Design review of the part built by this model. Coordinates are the model's own, in mm. A direction names the side the tool comes from. Coordinates: 2 decimals unless noted, no trailing zeros.
Q1. Add section A-A on x = 18.5. Give the number of separate pieces and of enclosed holes in the cut face, and give its area (3 significant figures).
Q2. Draft analysis for pull direction X (two halves, no side actions). For faces 1 (the face through (-26.453, -25.269, 5.07)), 2 (the face through (14, 1, 10)), 3 (the face through (60, 1, 5)), state which applies: released by +X, released by -X, zero draft, split by the parting line, or undercut.
Q3. Machinability: for faces 4 (the face through (15.894, 29.056, 5.07)), 5 (the face through (-60, -1, 5)), which of the approach directions +Z, -Z, +X, -X, +Y, -Y give a long, thin tool a straight path to every point of the face, cutting with its end or side? Answer none if there is none.
Q4. Wall thickness on probe 1 along Y at (x, z) = (-21, 3.5); probe 2 along Y at (x, z) = (-22, 8); probe 3 along Y at (x, z) = (-8, 8): over which ranges is each line inside the solid? List them lowest first.
```python
from build123d import *

# Parameters (mm, degrees)
BOSS_EXTRUDE1_DEPTH = 10
CUT_EXTRUDE32_DEPTH = 10


with BuildPart() as part:
    # Sketch1 → Boss-Extrude1 (new body)
    with BuildSketch(Plane.XY):
        with BuildLine():
            Line((-50, 60), (50, 60))
            ThreePointArc((50, 60), (57.071067812, 57.071067812), (60, 50))
            Line((60, 50), (60, -50))
            ThreePointArc((60, -50), (57.071067812, -57.071067812), (50, -60))
            Line((50, -60), (-50, -60))
            ThreePointArc((-50, -60), (-57.071067812, -57.071067812), (-60, -50))
            Line((-60, -50), (-60, 50))
            ThreePointArc((-60, 50), (-57.071067812, 57.071067812), (-50, 60))
        make_face()
    extrude(amount=BOSS_EXTRUDE1_DEPTH)

    # Sketch2 → Cut-Extrude32 (cut)
    with BuildSketch(Plane.XY.offset(10)):
        with BuildLine():
            Line((22.179487179, 34.806690705), (9.429086538, 23.141025641))
            add(Edge.make_bspline(
                [(9.429086538, 23.141025641), (8.882914048, 23.91145872), (7.834339031, 25.390582792), (6.134708299, 27.371164786), (4.442752271, 29.06074862), (2.742796004, 30.452275993), (1.019771731, 31.537292342), (-0.723329628, 32.305495903), (-2.476625945, 32.793850197), (-3.654570423, 32.854662056), (-4.234775641, 32.884615385)],
                knots=[0, 0, 0, 0, 1.299362458, 2.494594718, 3.587462134, 4.587049575, 5.512617175, 6.380583204, 7.202344345, 8, 8, 8, 8], degree=3))
            add(Edge.make_bspline(
                [(-4.234775641, 32.884615385), (-4.775974426, 32.865635582), (-5.820887089, 32.828990568), (-7.31048761, 32.464741869), (-8.632976167, 31.836102106), (-9.787062069, 31.01410273), (-10.701268375, 30.023784052), (-11.431191215, 28.98519439), (-11.842199109, 27.838826287), (-11.896295835, 27.05145443), (-11.923076923, 26.661658654)],
                knots=[0, 0, 0, 0, 1.185010067, 2.2879431, 3.333075148, 4.379039566, 5.372662701, 6.27520591, 7.14612461, 8, 8, 8, 8], degree=3))
            add(Edge.make_bspline(
                [(-11.923076923, 26.661658654), (-11.906294573, 26.266241849), (-11.872497251, 25.469927355), (-11.546061132, 24.302829291), (-11.054028691, 23.162438622), (-10.583871606, 22.468228557), (-10.343549679, 22.11338141)],
                knots=[0, 0, 0, 0, 0.967525499, 1.948461899, 2.951351359, 4, 4, 4, 4], degree=3))
            add(Edge.make_bspline(
                [(-10.343549679, 22.11338141), (-10.125071051, 21.837562436), (-9.622162103, 21.202663585), (-8.663217741, 20.197082772), (-7.458985017, 18.965158257), (-5.96312252, 17.549252313), (-4.237727617, 15.898443424), (-2.202826025, 14.077625518), (0.083008913, 12.030409979), (1.707727428, 10.604803211), (2.559094551, 9.857772436)],
                knots=[0, 0, 0, 0, 0.473873513, 1.090794244, 1.870441696, 2.795289791, 3.865433203, 5.087734844, 6.473946851, 8, 8, 8, 8], degree=3))
            add(Edge.make_bspline(
                [(2.559094551, 9.857772436), (3.358225064, 9.166165286), (4.874808752, 7.853638601), (7.032606174, 5.990717711), (8.92895073, 4.31469321), (10.591467834, 2.85071864), (11.994955347, 1.583433555), (13.145313536, 0.506780349), (14.056592075, -0.358280522), (14.574600568, -0.880777815), (14.795673077, -1.103766026)],
                knots=[0, 0, 0, 0, 1.543621617, 2.929473131, 4.163658386, 5.240097082, 6.164993805, 6.925417477, 7.541396219, 8, 8, 8, 8], degree=3))
            add(Edge.make_bspline(
                [(14.795673077, -1.103766026), (15.634376084, -2.011422303), (17.246657803, -3.756256423), (19.342055672, -6.460200571), (21.066635897, -9.099801404), (22.400803862, -11.724727295), (23.40842117, -14.372850698), (24.118804721, -17.109116699), (24.544258155, -19.96211756), (24.59149342, -21.908942364), (24.615384615, -22.893629808)],
                knots=[0, 0, 0, 0, 1.206664779, 2.319633467, 3.337109185, 4.282041471, 5.190008762, 6.099243693, 7.03861361, 8, 8, 8, 8], degree=3))
            add(Edge.make_bspline(
                [(24.615384615, -22.893629808), (24.598379474, -23.853086961), (24.565014754, -25.735577605), (24.156360918, -28.490322254), (23.573644532, -31.126732441), (22.672662774, -33.616120296), (21.574551543, -35.999348361), (20.197910517, -38.239293521), (18.581234396, -40.358624937), (16.728275333, -42.319456968), (14.67868258, -44.098776126), (12.480299564, -45.682768067), (10.111629387, -46.990555178), (7.592909595, -48.06742458), (4.925488401, -48.896843793), (2.112543508, -49.509861892), (-0.850227675, -49.877785692), (-2.876213304, -49.91624776), (-3.911258013, -49.935897436)],
                knots=[0, 0, 0, 0, 1.043214005, 2.046824704, 3.02475056, 3.976699089, 4.921714032, 5.875962561, 6.831408892, 7.817874052, 8.806269674, 9.781291748, 10.760897367, 11.74438705, 12.757449933, 13.795994037, 14.874007457, 16, 16, 16, 16], degree=3))
            add(Edge.make_bspline(
                [(-3.911258013, -49.935897436), (-4.723759295, -49.921483122), (-6.332977804, -49.892934513), (-8.704722601, -49.659858889), (-10.994910313, -49.283699628), (-13.200961249, -48.74455104), (-15.332814058, -48.061376655), (-17.390556291, -47.226905315), (-19.359982672, -46.228203026), (-21.255994813, -45.085807078), (-23.069375756, -43.759334902), (-24.82305499, -42.275905787), (-26.499613308, -40.612703931), (-28.107102878, -38.773662739), (-29.635238535, -36.753574491), (-31.134041642, -34.580572653), (-32.53690088, -32.214329262), (-33.403509434, -30.554390381), (-33.846153846, -29.706530449)],
                knots=[0, 0, 0, 0, 1.016823716, 2.013894106, 2.979844003, 3.91962641, 4.853723003, 5.779685073, 6.695824784, 7.614987388, 8.547259901, 9.504950863, 10.487499108, 11.500346958, 12.559593716, 13.656357062, 14.802919212, 16, 16, 16, 16], degree=3))
            Line((-33.846153846, -29.706530449), (-18.850160256, -20.705128205))
            add(Edge.make_bspline(
                [(-18.850160256, -20.705128205), (-18.296478254, -21.667560008), (-17.235022533, -23.512624029), (-15.436286582, -25.991701389), (-13.593573429, -28.114620785), (-11.664281196, -29.843859481), (-9.671869355, -31.202539621), (-7.606714094, -32.173546708), (-5.467364474, -32.774598996), (-4.010136703, -32.848001363), (-3.283253205, -32.884615385)],
                knots=[0, 0, 0, 0, 1.283663364, 2.460892379, 3.537111102, 4.529833553, 5.449777664, 6.316464042, 7.160231139, 8, 8, 8, 8], degree=3))
            add(Edge.make_bspline(
                [(-3.283253205, -32.884615385), (-2.543908622, -32.854714389), (-1.109472453, -32.796702103), (0.938001622, -32.26086011), (2.81520338, -31.41954887), (4.437842715, -30.219113746), (5.811791397, -28.83362916), (6.825844389, -27.292214207), (7.462879318, -25.624440438), (7.530229355, -24.465895073), (7.564102564, -23.883213141)],
                knots=[0, 0, 0, 0, 1.13588714, 2.203786484, 3.234766741, 4.283437687, 5.291419208, 6.222934724, 7.106237994, 8, 8, 8, 8], degree=3))
            add(Edge.make_bspline(
                [(7.564102564, -23.883213141), (7.532822042, -23.341122423), (7.469278655, -22.239917025), (7.001237654, -20.602601675), (6.26954681, -18.966030942), (5.403904944, -17.62367135), (4.523005953, -16.499750052), (3.68066783, -15.525923088), (2.654922822, -14.450014779), (1.448371765, -13.270671713), (0.076956347, -11.977511836), (-1.460478671, -10.570661777), (-3.181538547, -9.062514205), (-4.397987064, -8.035178979), (-5.034054487, -7.497996795)],
                knots=[0, 0, 0, 0, 0.916159276, 1.861089862, 2.860218735, 3.940849679, 4.552606315, 5.27541173, 6.11797699, 7.06649574, 8.129236253, 9.306560635, 10.591630461, 12, 12, 12, 12], degree=3))
            add(Edge.make_bspline(
                [(-5.034054487, -7.497996795), (-6.243243975, -6.474906536), (-8.564044597, -4.511286663), (-11.84363032, -1.611081927), (-14.798830707, 1.099425143), (-17.404121473, 3.653742339), (-19.692698053, 6.004697341), (-21.649061212, 8.171385505), (-23.251719411, 10.170519868), (-24.938171589, 12.538360741), (-26.540638342, 15.423737543), (-27.925624358, 18.895180326), (-28.824144829, 22.366182634), (-28.924811551, 24.696422404), (-28.974358974, 25.843349359)],
                knots=[0, 0, 0, 0, 1.345494975, 2.582412109, 3.71882943, 4.751509156, 5.681369928, 6.505683931, 7.230279997, 7.856715994, 8.973648664, 10.023341002, 11.027102913, 12, 12, 12, 12], degree=3))
            add(Edge.make_bspline(
                [(-28.974358974, 25.843349359), (-28.953752267, 26.656688395), (-28.91315484, 28.259053664), (-28.551019527, 30.61509832), (-28.009794504, 32.888483451), (-27.223780391, 35.070914712), (-26.203628979, 37.159658519), (-24.964694716, 39.164940152), (-23.487739299, 41.068303453), (-21.823310254, 42.868486626), (-19.989535587, 44.513649186), (-18.029914316, 45.965669991), (-15.955538071, 47.192067876), (-13.779096835, 48.209453974), (-11.487104107, 48.988198402), (-9.096444894, 49.540211269), (-6.60369023, 49.868530918), (-4.908172315, 49.913162165), (-4.044471154, 49.935897436)],
                knots=[0, 0, 0, 0, 1.010766082, 1.991317756, 2.957454644, 3.913069143, 4.869106762, 5.843196583, 6.838735724, 7.860187025, 8.887984031, 9.89767229, 10.887916223, 11.879572884, 12.879850636, 13.892031539, 14.926195476, 16, 16, 16, 16], degree=3))
            add(Edge.make_bspline(
                [(-4.044471154, 49.935897436), (-2.925157197, 49.894950547), (-0.695364756, 49.813379988), (2.601447679, 49.175524879), (5.821636228, 48.17243053), (8.416524509, 46.962307558), (10.481228679, 45.790060863), (12.063631555, 44.71080377), (13.673811657, 43.474456765), (15.324754087, 42.07712379), (16.98578178, 40.492477259), (18.704125696, 38.758240928), (20.456371299, 36.85942694), (21.595053116, 35.502923032), (22.179487179, 34.806690705)],
                knots=[0, 0, 0, 0, 1.282922637, 2.555718331, 3.837320111, 5.142675274, 5.830281639, 6.55870424, 7.337177975, 8.157850921, 9.037902056, 9.96903443, 10.957596896, 12, 12, 12, 12], degree=3))
        make_face()
    extrude(amount=-CUT_EXTRUDE32_DEPTH, mode=Mode.SUBTRACT)


solid = part.part
```
Entries:
1. separate pieces: 3
1. enclosed holes: 0
1. area: 775 mm2
2. face 1: undercut
2. face 2: zero draft
2. face 3: released by +X
3. face 4: +Z, -Z
3. face 5: +Z, -Z, -X, +Y, -Y
4. probe 1: y = -60 to -45.21, -22 to 7.47, 43.59 to 60
4. probe 2: y = -60 to -44.53, -22.6 to 8.63, 42.64 to 60
4. probe 3: y = -60 to -49.72, -31.95 to -4.98, 19.52 to 32.12, 49.67 to 60
